Check sheet for the modelled part. Datum: model origin and axes. Units: mm. A direction names the side the tool comes from. Give positions to 0.01 mm unless a question says otherwise; leave off trailing zeros. Write each loop counter-clockwise with the first axis right and the second up, starting at its lowest first coordinate (ties: lowest second). Pieces come first, ordered by that corner, then holes. Notation, with made-up numbers: (75.25, -8) - (89.25, -8) arc R22 ccw to (89.25, 2) - close; hole circle Ø10 at (66.5, 56.5). An arc over 180 degrees is marked (long way). Return JSON: item names as keys, results as strings. Group by question number.
```python
from build123d import *

# Parameters (mm, degrees)
SKETCH1_R                                       = 9.525
BOSS_EXTRUDE1_DEPTH                             = 34.925
SKETCH2_R                                       = 25.4
BOSS_EXTRUDE2_DEPTH                             = 3.175
SKETCH3_R                                       = 4.7625
BOSS_EXTRUDE3_DEPTH                             = 12.7
SKETCH4_R                                       = 2.15265
CUT_EXTRUDE1_DEPTH                              = 19.05
CIRPATTERN1_COUNT                               = 8
FILLET1_R                                       = 3
F_16_6MMFORKEYWAYDEPTHAND_6MMFOREXTRA_375_DEPTH = 17.1500038


with BuildPart() as part:
    # Sketch1 → Boss-Extrude1 (new body)
    with BuildSketch(Plane.XY):
        Circle(SKETCH1_R)
    extrude(amount=BOSS_EXTRUDE1_DEPTH)

    # Sketch2 → Boss-Extrude2 (add)
    with BuildSketch(Plane.XY.offset(34.925)):
        Circle(SKETCH2_R)
    extrude(amount=BOSS_EXTRUDE2_DEPTH)

    # Sketch3 → Boss-Extrude3 (add)
    with BuildSketch(Plane.XY.offset(38.1)):
        Circle(SKETCH3_R)
    extrude(amount=BOSS_EXTRUDE3_DEPTH)

    # Sketch4 → Cut-Extrude1 (cut)
    with BuildSketch(Plane.XY.offset(38.1)):
        with Locations((0, 19.05)):
            Circle(SKETCH4_R)
    cut_extrude1 = extrude(amount=-CUT_EXTRUDE1_DEPTH, mode=Mode.SUBTRACT)

    # CirPattern1: Cut-Extrude1 ×8 about axis
    cirpattern1_axis = Axis((0, 0, 0), (0, 0, 1))
    for i in range(1, CIRPATTERN1_COUNT):
        add(cut_extrude1.rotate(cirpattern1_axis, i * 360 / CIRPATTERN1_COUNT), mode=Mode.SUBTRACT)

    # Fillet1
    fillet1_edges = [part.edges().sort_by_distance(p)[0] for p in [
        (-4.7625, 0, 38.1),
    ]]
    fillet(fillet1_edges, radius=FILLET1_R)

    # Sketch5 → 16.6mmForKeywayDepthand.6mmForExtra.375 (cut)
    with BuildSketch(Plane(origin=(0, 0, 0), x_dir=(-1, 0, 0), z_dir=(0, 0, -1))):
        with BuildLine():
            Line((-1.5, 5.2), (1.5, 5.2))
            Line((1.5, 5.2), (1.5, 3.708099244))
            ThreePointArc((1.5, 3.708099244), (0, -4), (-1.5, 3.708099244))
            Line((-1.5, 3.708099244), (-1.5, 5.2))
        make_face()
    extrude(amount=-F_16_6MMFORKEYWAYDEPTHAND_6MMFOREXTRA_375_DEPTH, mode=Mode.SUBTRACT)


solid = part.part
```
Item 1: Depth check by flat-ended pin: pin 1 (3 mm diameter, centred on y = 4, z = 39, fed in from -X); pin 2 (2 mm diameter, centred on x = -12, y = 9, fed in from -Z) (3 decimals); pin 3 (1 mm diameter, centred on x = -9, z = 11.5, fed in from -Y); pin 4 (4 mm diameter, centred on x = 19.05, y = 0, fed in from -Z) (1 decimal). Enter the tip coordinate at first touch or a pass-through.
Item 2: Access from +Z, -Z, +X, -X, +Y, -Y to the whole of each face (thin tool, end or side, straight path). Record for faces 1 (the face through (-15.38, -12.48, 36.53)), 2 (the face through (0, 1, 17.15)), 3 (the face through (-3.78, -2.9, 45.88)).
Item 3: Material ranges on line 1 along Y through (x, z) = (0, 35.65); line 2 along X through (y, z) = (-1.5, 38); line 3 along Z through (x, y) = (-2, 23) (3 decimals), recorded low to high. Write a range as from..to.
Item 4: Section check A-A on y = 0. Count the separate pieces of the cut face and the enclosed holes in it, plus the area to 3 significant figures.
Item 5: Mould release check, pull along Y, two halves, no side actions. Record for faces 4 (the face through (-5.506, -24.796, 36.49)), 5 (the face through (5.3, 6, 38.1)), 6 (the face through (21.184, 0.28, 36.535)): +Y half, -Y half, draft (parallel to the pull), parting line (faces both ways), or undercut.
Item 6: Section check C-C on y = 19.05. Record the cut outline in (x, z) (3 decimals), plus the area to 3 significant figures.
Reply:
{
 "1": {"pin 1": "x = -25.25", "pin 2": "z = 34.925", "pin 3": "y = -4.3", "pin 4": "through"},
 "2": {"face 1": "+Z, -Z", "face 2": "-Z", "face 3": "+Z"},
 "3": {"line 1": "-25.4..-21.2, -16.9..16.9, 21.2..25.4", "line 2": "-25.36..-20.59, -17.51..17.51, 20.59..25.36", "line 3": "34.925..38.1"},
 "4": {"separate pieces": "3", "enclosed holes": "0", "area": "787 mm²"},
 "5": {"face 4": "parting line", "face 5": "draft", "face 6": "undercut"},
 "6": {"outline": "(-16.801, 34.925) - (-2.153, 34.925) - (-2.153, 38.1) - (-16.801, 38.1) - close; (2.153, 34.925) - (16.801, 34.925) - (16.801, 38.1) - (2.153, 38.1) - close", "area": "93.0 mm²"}
}
